Could you check a few things on this model? Use its own coordinates, in mm. A direction names the side the tool comes from. Coordinates: 2 decimals unless noted, no trailing zeros. Loops run counter-clockwise (first coordinate to the right, second up) from the corner with the lowest first, then second, coordinate; pieces in that order, holes last.
from build123d import *

# Parameters (mm, degrees)
F1_DEPTH = 32
F2_R     = 5.5
F3_DEPTH = 25
F4_R     = 6.5
F5_DEPTH = 132.41419


with BuildPart() as f1:
    # F0 (on Front) → F1 (new body)
    with BuildSketch(Plane.XZ):
        Polygon((0, 13), (0, 0), (39, 0), (39, 17), (74, 17), (74, 0), (113, 0), (113, 13), (88, 13), (88, 64), (69, 64), (69, 30), (44, 30), (44, 64), (25, 64), (25, 13), align=None)
    extrude(amount=F1_DEPTH)

    # F2 (on Top) → F3 (cut)
    with BuildSketch(Plane.XY):
        with Locations((13, -13)):
            Circle(F2_R)
        with Locations((100, -13)):
            Circle(F2_R)
        Polygon((10, -32), (0, -22), (0, -32), align=None)
        Polygon((113, -22), (103, -32), (113, -32), align=None)
    extrude(amount=F3_DEPTH, mode=Mode.SUBTRACT)

    # F4 (on Right) → F5 (cut)
    with BuildSketch(Plane.YZ):
        with Locations((-16, 46)):
            Circle(F4_R)
        with BuildLine():
            ThreePointArc((-32, 61.440635), (-15.948352, 63.505935), (0, 60.7544))
            Line((0, 60.7544), (0, 64))
            Line((0, 64), (-32, 64))
            Line((-32, 64), (-32, 61.440635))
        make_face()
    extrude(amount=F5_DEPTH, mode=Mode.SUBTRACT)


solid = f1.part
(1) For pin 1 (16 mm diameter, centred on y = -13, z = 43.5, fed in from +X); pin 2 (3 mm diameter, centred on x = 57, z = 25.5, fed in from +Y); pin 3 (8 mm diameter, centred on y = -6.5, z = 50, fed in from -X); pin 4 (7.5 mm diameter, centred on x = 18.5, y = -21, fed in from +Z), each with a flat end and sliding along its axis, tell me the tip position at first contact or that it passes through.
Answers:
pin 1: stops at x = 88
pin 2: stops at y = 0
pin 3: stops at x = 25
pin 4: stops at z = 13
(2) Imagine slicing it at A-A, the plane z = 46. Write out the boundary of the cut face in (x, y).
Answers:
outline: (25, -32) - (44, -32) - (44, -22.5) - (25, -22.5) - close; (25, -9.5) - (44, -9.5) - (44, 0) - (25, 0) - close; (69, -32) - (88, -32) - (88, -22.5) - (69, -22.5) - close; (69, -9.5) - (88, -9.5) - (88, 0) - (69, 0) - close
(3) We'd pull the mould along Y, two halves only. Please class faces 6 (the face through (18.08, -15.11, 6.41)), 7 (the face through (19, -16, 0)), 8 (the face through (66, -32, 24)), 9 (the face through (94.505, -12.758, 6.409)): +Y half, -Y half, draft (parallel to the pull), parting line (faces both ways), or undercut.
Answers:
face 6: undercut
face 7: draft
face 8: -Y half
face 9: undercut
(4) Which directions (+Z, -Z, +X, -X, +Y, -Y) give clear straight access to the entire face, cutting with the end or side of a thin tool? Please do faces 1 (the face through (69, -23, 47)), 2 (the face through (74, -16, 9)), 3 (the face through (56, 0, 24)), 4 (the face through (13, -19, 13)), 5 (the face through (88, -16, 38)).
Answers:
face 1: +Z, +Y, -Y
face 2: -Z, +Y, -Y
face 3: +Z, -Z, +X, -X, +Y
face 4: +Z, -X, +Y, -Y
face 5: +Z, +X, +Y, -Y
(5) I need wall thicknesses on probe 1 along X at (y, z) = (-16, 60); probe 2 along Y at (x, z) = (100, 4.25); probe 3 along X at (y, z) = (-13, 4). Which ranges of each line are inside material? Lowest first, please.
Answers:
probe 1: x = 25 to 44, 69 to 88
probe 2: y = -32 to -18.5, -7.5 to 0
probe 3: x = 0 to 7.5, 18.5 to 39, 74 to 94.5, 105.5 to 113
(6) Imagine slicing it at B-B, the plane x = 100. Write out the boundary of the cut face in (y, z), and give its area (3 significant figures).
Answers:
outline: (-32, 0) - (-18.5, 0) - (-18.5, 13) - (-32, 13) - close; (-7.5, 0) - (0, 0) - (0, 13) - (-7.5, 13) - close
area: 273 mm2
(7) Imagine slicing it at C-C, the plane z = 35.5. Write out the boundary of the cut face in (x, y).
Answers:
outline: (25, -32) - (44, -32) - (44, 0) - (25, 0) - close; (69, -32) - (88, -32) - (88, 0) - (69, 0) - close
(8) Imagine slicing it at D-D, the plane x = 80.5. Write out the boundary of the cut face in (y, z), and give its area (3 significant figures).
Answers:
outline: (-32, 0) - (0, 0) - (0, 60.75) arc R54.36 ccw to (-32, 61.44) - close; hole circle Ø13 at (-16, 46)
area: 1,870 mm2
